For this review, take the finished solid that the model builds, in its own axes (mm). A direction names the side the tool comes from. Coordinates: 2 decimals unless noted, no trailing zeros. Loops run counter-clockwise (first coordinate to the right, second up) from the corner with the lowest first, then second, coordinate; pieces in that order, holes last. Notation, with made-up numbers: M 35,57 L 71,57 A16 ccw 71,79 Z; hole C -15.75,53 d2. An arc over 180 degrees is marked long. Use one line per item in the form item = value.
```python
from build123d import *

# Parameters (mm, degrees)
SKETCH1_R           = 98
SKETCH1_R_2         = 5
BOSS_EXTRUDE1_DEPTH = 10
SKETCH2_W           = 65
SKETCH2_H           = 65
BOSS_EXTRUDE2_DEPTH = 50
SKETCH3_W           = 120
SKETCH3_H           = 65
SKETCH3_R           = 5
BOSS_EXTRUDE3_DEPTH = 6
SKETCH4_W           = 45
SKETCH4_H           = 45
CUT_EXTRUDE1_DEPTH  = 154.50570022


with BuildPart() as part:
    # Sketch1 → Boss-Extrude1 (new body)
    with BuildSketch(Plane(origin=(0, 0, 0), x_dir=(1, 0, 0), z_dir=(0, 1, 0))):
        with Locations(Location((0, 0, 0), (0, 0, 270))):
            Circle(SKETCH1_R)
        with Locations(Location((0, 90, 0), (0, 0, 270))):
            Circle(SKETCH1_R_2, mode=Mode.SUBTRACT)
        with Locations(Location((85.595086467, 27.811529494, 0), (0, 0, 270))):
            Circle(SKETCH1_R_2, mode=Mode.SUBTRACT)
        with Locations(Location((52.900672706, -72.811529494, 0), (0, 0, 270))):
            Circle(SKETCH1_R_2, mode=Mode.SUBTRACT)
        with Locations(Location((-52.900672706, -72.811529494, 0), (0, 0, 270))):
            Circle(SKETCH1_R_2, mode=Mode.SUBTRACT)
        with Locations(Location((-85.595086467, 27.811529494, 0), (0, 0, 270))):
            Circle(SKETCH1_R_2, mode=Mode.SUBTRACT)
    extrude(amount=BOSS_EXTRUDE1_DEPTH)

    # Sketch2 → Boss-Extrude2 (add)
    with BuildSketch(Plane(origin=(0, 10, 0), x_dir=(1, 0, 0), z_dir=(0, 1, 0))):
        Rectangle(SKETCH2_W, SKETCH2_H)
    extrude(amount=BOSS_EXTRUDE2_DEPTH)

    # Sketch3 → Boss-Extrude3 (add)
    with BuildSketch(Plane(origin=(0, 60, 0), x_dir=(1, 0, 0), z_dir=(0, 1, 0))):
        Rectangle(SKETCH3_W, SKETCH3_H)
        with Locations(Location((-46.25, 16.25, 0), (0, 0, 270))):
            Circle(SKETCH3_R, mode=Mode.SUBTRACT)
        with Locations(Location((46.25, 16.25, 0), (0, 0, 90))):
            Circle(SKETCH3_R, mode=Mode.SUBTRACT)
        with Locations(Location((46.25, -16.25, 0), (0, 0, 270))):
            Circle(SKETCH3_R, mode=Mode.SUBTRACT)
        with Locations(Location((-46.25, -16.25, 0), (0, 0, 90))):
            Circle(SKETCH3_R, mode=Mode.SUBTRACT)
    extrude(amount=BOSS_EXTRUDE3_DEPTH)

    # Sketch4 → Cut-Extrude1 (cut, through all)
    with BuildSketch(Plane(origin=(0, 66, 0), x_dir=(1, 0, 0), z_dir=(0, 1, 0))):
        Rectangle(SKETCH4_W, SKETCH4_H)
    extrude(amount=-CUT_EXTRUDE1_DEPTH, mode=Mode.SUBTRACT)


solid = part.part
```
1. Wall thickness on line 1 along X through (y, z) = (64, -16); line 2 along Z through (x, y) = (45.5, 60.5); line 3 along X through (y, z) = (26, 8): over which ranges is each line inside the solid? List them lowest first. Write a range as from..to.
Computed values:
line_1 = -60..-51.24, -41.26..-22.5, 22.5..41.26, 51.24..60
line_2 = -32.5..-21.19, -11.31..11.31, 21.19..32.5
line_3 = -32.5..-22.5, 22.5..32.5
2. Consider section C-C on x = 35. Write out the cut boundary in (y, z).
Computed values:
outline = M 0,-91.54 L 10,-91.54 L 10,91.54 L 0,91.54 Z; M 60,-32.5 L 66,-32.5 L 66,32.5 L 60,32.5 Z
3. Consider section B-B on z = 0. Write out the cut boundary in (x, y), plus the area to 3 significant figures.
Computed values:
outline = M -98,0 L -22.5,0 L -22.5,66 L -60,66 L -60,60 L -32.5,60 L -32.5,10 L -98,10 Z; M 22.5,0 L 98,0 L 98,10 L 32.5,10 L 32.5,60 L 60,60 L 60,66 L 22.5,66 Z
area = 2,960 mm2
4. Draft analysis for pull direction X (two halves, no side actions). For faces 1 (the face through (1, 10, 42)), 2 (the face through (0, 33, -22.5)), 3 (the face through (-32.5, 35, 0)), state which applies: +X half, -X half, draft (parallel to the pull), parting line (faces both ways), or undercut.
Computed values:
face_1 = draft
face_2 = undercut
face_3 = -X half
5. For pin 1 Ø1.5 at (x, z) = (75.5, 35.5) entering from +Y; pin 2 Ø6 at (x, z) = (0, -90) entering from -Y; pin 3 Ø17 at (x, y) = (-20, 35) entering from +Z; pin 4 Ø6 at (x, y) = (-29.5, 36) entering from -Z, all flat-tipped, find the tip position at first contact; note any pin that passes through.
Computed values:
pin_1 = 10
pin_2 = through
pin_3 = 32.5
pin_4 = -32.5
6. Tool access review of faces 4 (the face through (-51.207, 62.958, 16.901)), 5 (the face through (60, 63, 0)), 6 (the face through (0, 33, 22.5)): name each direction out of +Z, -Z, +X, -X, +Y, -Y from which nothing blocks a thin tool from reaching the whole face with its end or side.
Computed values:
face_4 = +Y
face_5 = +Z, -Z, +X, +Y
face_6 = +Y, -Y
7. Consider section A-A on y = 53.5. Write out the cut boundary in (x, z), plus the area to 3 significant figures.
Computed values:
outline = M -32.5,-32.5 L 32.5,-32.5 L 32.5,32.5 L -32.5,32.5 Z; hole M -22.5,-22.5 L 22.5,-22.5 L 22.5,22.5 L -22.5,22.5 Z
area = 2,200 mm2
8. Consider section D-D on z = -90. Write out the cut boundary in (x, y), plus the area to 3 significant figures.
Computed values:
outline = M -38.78,0 L -5,0 L -5,10 L -38.78,10 Z; M 5,0 L 38.78,0 L 38.78,10 L 5,10 Z
area = 676 mm2
